Autodesk Inventor part; units mm, degrees
ref_plane "YZ Plane" through (0, 0, 0) normal (1, 0, 0) x (0, 1, 0)
ref_plane "XZ Plane" through (0, 0, 0) normal (0, 1, 0) x (-1, 0, 0)
ref_plane "XY Plane" through (0, 0, 0) normal (0, 0, 1) x (1, 0, 0)
sketch "Sketch1" plane through (0, 0, 0) normal (0, 1, 0) x (-1, 0, 0)
  point P0 (0, 0)
sketch "Sketch2" plane through (0, 0, 0) normal (0, 1, 0) x (-1, 0, 0)
  line L0 (0, 0) -> (28.2, 0)
  line L1 (28.2, 0) -> (28.2, -28.2)
  line L2 (28.2, -28.2) -> (0, -28.2)
  line L3 (0, -28.2) -> (0, 0)
  dimension "d0" = 28.2
  dimension "d1" = 28.2
extrude "Extrusion1" add sketch "Sketch2" along normal blind 32
sketch "Sketch3" plane through (0, 32, 0) normal (0, 1, 0) x (1, 0, 0)
  circle A0 centre (-14.1, 14.1) radius 11
  point P0 (0, 0)
  dimension "d4" = 22
extrude "Extrusion2" add sketch "Sketch3" along normal blind 2
sketch "Sketch4" plane through (-14.1, 34, -14.1) normal (0, 1, 0) x (1, 0, 0)
  circle A0 centre (0, 0) radius 2.5
  point P0 (14.1, -14.1)
  dimension "d7" = 5
extrude "Extrusion3" add sketch "Sketch4" along normal blind 20
sketch "Sketch5" plane through (0, 32, 0) normal (0, 1, 0) x (1, 0, 0)
  circle A0 centre (-25.6, 2.6) radius 1.25
  line L0 (-28.2, 28.2) -> (-28.2, 0)
  line L1 (-28.2, 0) -> (0, 0)
  circle A1 centre (-25.6, 25.6) radius 1.25
  circle A2 centre (-2.6, 2.6) radius 1.25
  circle A3 centre (-2.6, 25.6) radius 1.25
  dimension "d10" = 2.5
  dimension "d11" = 2.6
  dimension "d12" = 2.6
  dimension "d13" = 2.5
  dimension "d14" = 23
  dimension "d15" = 2.5
  dimension "d16" = 23
  dimension "d17" = 2.5
extrude "Extrusion4" cut sketch "Sketch5" against normal through all
fillet "Fillet1" radius 2 4 edges at (0, 16, 0) (0, 16, -28.2) (-28.2, 16, -28.2) (-28.2, 16, 0)
properties part number "NEMA11"
Could you check a few things on this model? Use its own coordinates, in mm. A direction names the side the tool comes from. Give positions to 0.01 mm unless a question says otherwise; leave off trailing zeros. Order: outer loops, then holes, each group sorted by start corner. A loop starts at its lowest first (then second) coordinate and runs counter-clockwise, first axis right, second up. Notation, with made-up numbers: (46, 48) - (81, 48) arc R17 cw to (81, 66) - close; hole circle Ø1 at (37, -7.75). An arc over 180 degrees is marked (long way). Return JSON: item names as keys, results as strings. Group by question number.
Q1. Thinking about a two-plate mould opening in X: for faces 1 (the face through (-26.521, 16.224, -26.445)), 2 (the face through (-14, 16, 0)), 3 (the face through (-22.21, 32.99, -6.67)), which applies, pulls with the +X half, pulls with the -X half, needs draft (parallel to the pull), parting line crosses it, or undercut?
Q2. Suppose I cut it at B-B, the plane x = -13.75. Please give me the cut outline in (y, z).
Q3. Suppose I cut it at A-A, the plane y = 6.5. Please give me the cut outline in (x, z), and give its area (3 significant figures).
Q4. Which directions (+Z, -Z, +X, -X, +Y, -Y) give clear straight access to the entire face, cutting with the end or side of a thin tool? Please do faces 4 (the face through (-4.5, 32, -7.6)), 5 (the face through (0, 16, -14)).
Q5. Suppose I cut it at D-D, the plane x = -20.5. Please give me the cut outline in (y, z), and give its area (3 significant figures).
Q6. Suppose I cut it at C-C, the plane z = -19.25. Please give me the cut outline in (x, y).
Q7. Please list where these lines run through material, in increasing order: line 1 along X through (y, z) = (22.5, -2.6); line 2 along Z through (x, y) = (-26.5, 20). Write a range as [from, to].
Q8. Will these pins go through, and if not, where does the flat tip stop? pin 1 Ø2 at (x, z) = (-2.6, -2.6) entering from +Y; pin 2 Ø4 at (x, z) = (-25.6, -2.6) entering from +Y; pin 3 Ø1.5 at (x, z) = (-10, -4.5) entering from +Y.
Resolved:
{
 "1": {"face 1": "undercut", "face 2": "needs draft", "face 3": "parting line crosses it"},
 "2": {"outline": "(0, -28.2) - (32, -28.2) - (32, -25.09) - (34, -25.09) - (34, -16.58) - (54, -16.58) - (54, -11.62) - (34, -11.62) - (34, -3.11) - (32, -3.11) - (32, 0) - (0, 0) - close"},
 "3": {"outline": "(-28.2, -26.2) arc R2 ccw to (-26.2, -28.2) - (-2, -28.2) arc R2 ccw to (0, -26.2) - (0, -2) arc R2 ccw to (-2, 0) - (-26.2, 0) arc R2 ccw to (-28.2, -2) - close; hole circle Ø2.5 at (-25.6, -25.6); hole circle Ø2.5 at (-25.6, -2.6); hole circle Ø2.5 at (-2.6, -25.6); hole circle Ø2.5 at (-2.6, -2.6)", "area": "772 mm2"},
 "4": {"face 4": "+Y", "face 5": "+Z, -Z, +X, +Y, -Y"},
 "5": {"outline": "(0, -28.2) - (32, -28.2) - (32, -23.05) - (34, -23.05) - (34, -5.15) - (32, -5.15) - (32, 0) - (0, 0) - close", "area": "938 mm2"},
 "6": {"outline": "(-28.2, 0) - (0, 0) - (0, 32) - (-4.38, 32) - (-4.38, 34) - (-23.82, 34) - (-23.82, 32) - (-28.2, 32) - close"},
 "7": {"line 1": "x = [-28.2, -26.85], [-24.35, -3.85], [-1.35, 0]", "line 2": "z = [-28.18, -26.47], [-24.73, -3.47], [-1.73, -0.02]"},
 "8": {"pin 1": "passes through", "pin 2": "stops at y = 32", "pin 3": "stops at y = 34"}
}
